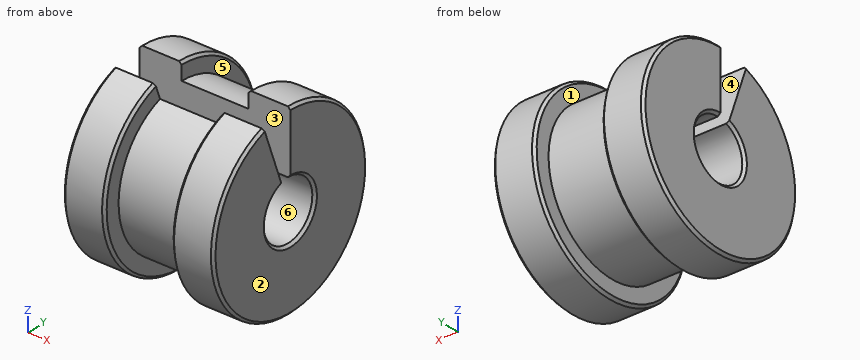
Autodesk Inventor part; units mm, degrees
ref_plane "YZ Plane" through (0, 0, 0) normal (1, 0, 0) x (0, 1, 0)
ref_plane "XZ Plane" through (0, 0, 0) normal (0, 1, 0) x (-1, 0, 0)
ref_plane "XY Plane" through (0, 0, 0) normal (0, 0, 1) x (1, 0, 0)
sketch "Sketch1" plane through (0, 0, 0) normal (0, 1, 0) x (-1, 0, 0)
  line L0 (-9, 0) -> (9, 0)
  line L1 (-9, 3.5) -> (9, 3.5)
  line L2 (9, 3.5) -> (9, 11)
  line L3 (9, 11) -> (4, 11)
  line L4 (4, 11) -> (4, 9)
  line L5 (4, 9) -> (-4, 9)
  line L6 (-4, 9) -> (-4, 11)
  line L7 (-4, 11) -> (-9, 11)
  line L8 (-9, 11) -> (-9, 3.5)
  point P0 (0, 0)
  point P1 (0, 9)
  point P2 (0, 3.5)
  dimension "d0" = 18
  dimension "d1" = 8
  dimension "d2" = 7
  dimension "d3" = 22
  dimension "d4" = 2
revolve "Revolution1" add sketch "Sketch1" angle 340 about axis through (9, 0, 0) along (-1, 0, 0)
chamfer "Chamfer1" distance 0.3 angle 45 6 edges at (-4, 1.9101, -10.8329) (4, 1.9101, -10.8329) (9, 1.9101, -10.8329) (-9, 1.9101, -10.8329) (9, 0.6078, -3.4468) (-9, 0.6078, -3.4468)
properties part number "coupling_tie" material "ABS Plastic"
Model file for the job. Use its own axes, mm. Face numbers are marked on the shaded views. A direction names the side the tool comes from. Give positions to 0.01 mm unless a question says otherwise; leave off trailing zeros. Order: outer loops, then holes, each group sorted by start corner. A loop starts at its lowest first (then second) coordinate and runs counter-clockwise, first axis right, second up.
1) Pin check, flat tips, straight feed: pin 1 (2 mm diameter, centred on x = 5, y = -3.5, fed in from +Z); pin 2 (2.5 mm diameter, centred on x = 3, z = 8, fed in from -Y); pin 3 (1 mm diameter, centred on x = -1, y = -5, fed in from -Z). Stop position of each tip, or through.
2) 3-axis set-ups, long thin cutter, end or side, ignore diameter. For the marked faces 4, 5 and 6: which of +Z, -Z, +X, -X, +Y, -Y reach the whole face in a straight line?
3) Wall check: probe 1 along Y at (x, z) = (1.5, 0); probe 2 along X at (y, z) = (4.25, -8); probe 3 along Y at (x, z) = (5.25, -2.5). Give the ranges that are in metal, low to high.
4) Saw through at B-B, the plane z = 9.75. Count the separate pieces of the cut face and the enclosed holes in it, then the cut area to 3 significant figures.
5) Mould opens along X. For the marked faces 1, 2 and 3 say: +X half, -X half, draft (parallel to the pull), parting line (faces both ways), or undercut.
6) Saw through at C-C, the plane x = 0.5. Write the cut outline in (y, z).
7) Saw through at A-A, the plane z = 0. Write the cut outline in (x, y).
Computed:
1. pin 1: stops at z = 10.34
1. pin 2: stops at y = -7.87
1. pin 3: stops at z = -7.79
2. face 4: +Z, +X, -X
2. face 5: none
2. face 6: +X, -X
3. probe 1: y = -9 to -3.5, 3.5 to 9
3. probe 2: x = -9 to -4, 4 to 9
3. probe 3: y = -10.71 to -2.45, 2.45 to 10.71
4. separate pieces: 4
4. enclosed holes: 0
4. area: 65.6 mm2
5. face 1: undercut
5. face 2: +X half
5. face 3: draft
6. outline: (-3.08, 8.46) arc R9 ccw (long way) to (0, 9) - (0, 3.5) arc R3.5 cw (long way) to (-1.2, 3.29) - close
7. outline: (-9, -10.7) - (-8.7, -11) - (-4.3, -11) - (-4, -10.7) - (-4, -9) - (4, -9) - (4, -10.7) - (4.3, -11) - (8.7, -11) - (9, -10.7) - (9, -3.8) - (8.7, -3.5) - (-8.7, -3.5) - (-9, -3.8) - close; (-9, 3.8) - (-8.7, 3.5) - (8.7, 3.5) - (9, 3.8) - (9, 10.7) - (8.7, 11) - (4.3, 11) - (4, 10.7) - (4, 9) - (-4, 9) - (-4, 10.7) - (-4.3, 11) - (-8.7, 11) - (-9, 10.7) - close
